Verification items for the finished model (mm, model axes). A direction names the side the tool comes from. Give positions to 0.01 mm unless a question says otherwise; leave off trailing zeros. Write each loop counter-clockwise with the first axis right and the second up, starting at its lowest first coordinate (ties: lowest second). Pieces come first, ordered by that corner, then holes. Notation, with made-up numbers: (-29, -14) -> (-23, -14) arc R21 cw to (-23, 24) -> close; hole circle Ø5 at (-20, -40). An arc over 180 degrees is marked (long way). Answer as CSV lines item,"result". Start each with the question number.
1) Sectioned sample at D-D on x = -12.5. Record the cut outline in (y, z).
2) Sectioned sample at B-B on x = -19. Record the cut outline in (y, z).
3) Mould release check, pull along Z, two halves, no side actions. Record for faces 5 (the flat face through (-21, 7.518, -11)), 6 (the flat face through (-19, 4, -14.381)), 7 (the cylindrical face through (-24.169, 3.812, -20.165)): released by +Z, released by -Z, zero draft, split by the parting line, or undercut.
4) Gauge pin test, flat ends, axial feed: pin 1 Ø2 at (x, y) = (-24, 1) entering from +Z; pin 2 Ø4 at (x, y) = (-13.5, 2.5) entering from +Z; pin 3 Ø5 at (x, z) = (-11.7, -8.08) entering from +Y; pin 4 Ø5 at (x, z) = (-23.08, -8.08) entering from -Y. Record the tip position at first contact, or that the pin passes through.
5) Sectioned sample at C-C on y = 7. Record the cut outline in (x, z), and give its area (3 significant figures).
6) Sectioned sample at A-A on z = -20.25. Record the cut outline in (x, y).
7) Material ranges on L1, parallel to X at y = 6.5, z = -9.75; L2, parallel to Y at x = -21, z = -13; L3, parallel to X at y = 5.75, z = -7.5, recorded low to high.
8) Tool access check on faces 1 (the flat face through (-24, 3, -13.162)), 2 (the flat face through (-16.783, 4, -2)), 3 (the flat face through (-20.441, 4, -19)), 4 (the flat face through (-30, 4, -14.381)). Record the directions out of +Z, -Z, +X, -X, +Y, -Y that give a thin tool (end or side, any length) a straight path to the whole face; none if there is none.
Autodesk Inventor part; units mm, degrees
ref_plane "YZ Plane" through (0, 0, 0) normal (1, 0, 0) x (0, 1, 0)
ref_plane "XZ Plane" through (0, 0, 0) normal (0, 1, 0) x (-1, 0, 0)
ref_plane "XY Plane" through (0, 0, 0) normal (0, 0, 1) x (1, 0, 0)
sketch "Sketch1" plane through (0, 0, 0) normal (0, 1, 0) x (-1, 0, 0)
  line L0 (16.7831, -1.7829) -> (16.7831, -14.3813)
  line L1 (16.7831, -14.3813) -> (29.3815, -14.3813)
  line L2 (28.1623, -3.0021) -> (18.0023, -3.0021)
  line L3 (18.0023, -3.0021) -> (18.0023, -13.1621)
  line L4 (18.0023, -13.1621) -> (28.1623, -13.1621)
  line L5 (28.1623, -13.1621) -> (28.1623, -3.0021)
  line L6 (28.1623, -3.0021) -> (29.3815, -3.0021)
  line L7 (30.6007, -14.3813) -> (20.4407, -14.3813)
  line L8 (20.4407, -14.3813) -> (20.4407, -24.5413)
  line L9 (20.4407, -24.5413) -> (30.6007, -24.5413)
  line L10 (30.6007, -24.5413) -> (30.6007, -14.3813)
  line L11 (16.7831, -3.0021) -> (6.6231, -3.0021)
  line L12 (6.6231, -3.0021) -> (6.6231, -13.1621)
  line L13 (6.6231, -13.1621) -> (16.7831, -13.1621)
  line L14 (16.7831, -13.1621) -> (16.7831, -3.0021)
  line L15 (28.1623, -13.1621) -> (29.3815, -13.1621)
  line L16 (18.0023, -3.0021) -> (18.0023, -1.7829)
  line L17 (29.3815, -13.1621) -> (29.3815, -14.3813)
  line L18 (18.0023, -1.7829) -> (16.7831, -1.7829)
  line L19 (18.0023, -1.7829) -> (16.7831, -1.7829)
  circle A0 centre (25.5207, -19.4613) radius 1.524
  circle A1 centre (11.7031, -8.0821) radius 1.524
  point P0 (0, 0)
  dimension "d16" = 3.048
  dimension "d17" = 3.048
extrude "Extrusion1" add sketch "Sketch1" along normal blind 5.1308 contours L18 L16 L3 L4 L15 L17 L1 L0
sketch "Sketch2" plane through (0, 5.1308, 0) normal (0, 1, 0) x (1, 0, 0)
  line L0 (-16.7831, 14.3813) -> (-29.3815, 14.3813)
  line L1 (-16.7831, 14.3813) -> (-29.3815, 14.3813)
  line L2 (-29.3815, 14.3813) -> (-29.3815, 1.7884)
  line L3 (-29.3815, 1.7884) -> (-16.7831, 1.7884)
  line L4 (-16.7831, 1.7884) -> (-16.7831, 14.3813)
  circle A0 centre (-23.0823, 8.0848) radius 1.524
  point P0 (0, 0)
  dimension "d4" = 3.048
extrude "Extrusion2" add sketch "Sketch2" along normal blind 2.3876 contours L4 L3 L2 L0 | A0
hole "Hole1" at (-23.0823, 5.1308, -8.0848) direction (0, 1, 0) diameter 3.048 end through all
extrude "Extrusion3" add sketch "Sketch1" along normal blind 7.5184 contours L1 L7 L10 L9 L8 | A0
extrude "Extrusion4" add sketch "Sketch1" along normal blind 7.5184 contours L0 L13 L12 L11 | A1
hole "Hole2" at (-11.7031, 0, -8.0821) direction (0, 1, 0) diameter 3.048 end through all
hole "Hole3" at (-25.5207, 0, -19.4613) direction (0, 1, 0) diameter 3.048 end through all
properties part number "tab"
Ans:
1,outline,"(0, -13.16) -> (7.52, -13.16) -> (7.52, -9.38) -> (0, -9.38) -> close; (0, -6.78) -> (7.52, -6.78) -> (7.52, -3) -> (0, -3) -> close"
2,outline,"(0, -14.38) -> (7.52, -14.38) -> (7.52, -1.79) -> (5.13, -1.79) -> (5.13, -13.16) -> (0, -13.16) -> close"
3,face 5,"zero draft"
3,face 6,"released by -Z"
3,face 7,"undercut"
4,pin 1,"stops at z = -13.16"
4,pin 2,"stops at z = -3"
4,pin 3,"stops at y = 7.52"
4,pin 4,"stops at y = 5.13"
5,outline,"(-30.6, -24.54) -> (-20.44, -24.54) -> (-20.44, -14.38) -> (-16.78, -14.38) -> (-16.78, -13.16) -> (-6.62, -13.16) -> (-6.62, -3) -> (-16.78, -3) -> (-16.78, -1.79) -> (-29.38, -1.79) -> (-29.38, -14.38) -> (-30.6, -14.38) -> close; hole circle Ø3.05 at (-25.52, -19.46); hole circle Ø3.05 at (-23.08, -8.08); hole circle Ø3.05 at (-11.7, -8.08)"
5,area,"343 mm²"
6,outline,"(-30.6, 0) -> (-26.82, 0) -> (-26.82, 7.52) -> (-30.6, 7.52) -> close; (-24.22, 0) -> (-20.44, 0) -> (-20.44, 7.52) -> (-24.22, 7.52) -> close"
7,L1,"x = -29.38 to -6.62"
7,L2,"y = 5.13 to 7.52"
7,L3,"x = -29.38 to -24.49, -21.67 to -13.11, -10.29 to -6.62"
8,face 1,"+Z, -X, -Y"
8,face 2,"+Z, +X, +Y, -Y"
8,face 3,"-Z, +X, +Y, -Y"
8,face 4,"+Z, -X, +Y, -Y"
